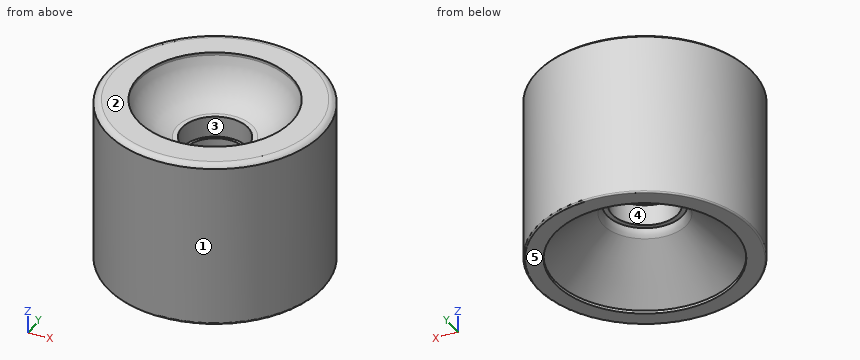
from build123d import *

# Parameters (mm, degrees)
FILLET1_R = 0.5


with BuildPart() as part:
    # Sketch1 → Revolve1 (revolve)
    with BuildSketch(Plane(origin=(0, 0, 0), x_dir=(1, 0, 0), z_dir=(0, 1, 0))):
        with BuildLine():
            Line((36, 56), (36, 1.160679473))
            ThreePointArc((36, 1.160679473), (34.94947687, 0.305750422), (33.63, 0))
            Line((33.63, 0), (25.63, 0))
            Line((25.63, 0), (25.63, 1))
            ThreePointArc((25.63, 1), (20.557422009, 8.606026819), (12.63, 13.16))
            Line((12.63, 13.16), (11, 13.16))
            Line((11, 13.16), (11, 20.16))
            Line((11, 20.16), (10, 20.16))
            Line((10, 20.16), (10, 30.16))
            Line((10, 30.16), (11, 30.16))
            Line((11, 30.16), (11, 37.16))
            Line((11, 37.16), (12.63, 37.16))
            ThreePointArc((12.63, 37.16), (12.964344278, 38.760927271), (13.911484064, 40.094224107))
            Line((13.911484064, 40.094224107), (30, 55))
            Line((30, 55), (30, 56))
            Line((30, 56), (36, 56))
        make_face()
    revolve(axis=Axis((0, 0, 0), (0, 0, -1)))

    # Fillet1
    fillet1_edges = [part.edges().sort_by_distance(p)[0] for p in [
        (-36, 0, -56),
    ]]
    fillet(fillet1_edges, radius=FILLET1_R)


solid = part.part
Here's how the part is built. I have some questions about the finished solid (model axes, mm). Face numbers are marked on the shaded views. A direction names the side the tool comes from. Give positions to 0.01 mm unless a question says otherwise; leave off trailing zeros. Order: outer loops, then holes, each group sorted by start corner. A loop starts at its lowest first (then second) coordinate and runs counter-clockwise, first axis right, second up. Notation, with made-up numbers: M 66.5,-23 L 111.5,-23 A10 ccw 111.5,-16 Z; hole C -24.5,36 d6. An arc over 180 degrees is marked long. Answer as a JSON object with one key per item and string values. Group by question number.
1) We'd pull the mould along Y, two halves only. Please class the marked faces 1, 2 and 3: pulls with the +Y half, pulls with the -Y half, needs draft (parallel to the pull), parting line crosses it, or undercut.
2) Suppose I cut it at A-A, the plane z = -39. Write out the boundary of the cut face in (x, y), plus the area to 3 significant figures.
3) On a 3-axis mill with a long thin cutter (end or side, diameter ignored), from which of +Z, -Z, +X, -X, +Y, -Y can I reach the whole of each face in a straight line? I mean the marked faces 4 and 5. Say none if no direction works.
4) I'm going to push flat-ended pins straight in: pin 1 Ø1.5 at (y, z) = (4, -13.5) entering from -X; pin 2 Ø12 at (y, z) = (18, -22.5) entering from +X; pin 3 Ø4 at (x, z) = (-19, -14) entering from +Y. Where does each tip first touch, or does it pass through?
5) Please list where these lines run through material, in increasing order: L1, parallel to Y at x = 0, z = -0.65; L2, parallel to Y at x = 0, z = -16. Write a range as [from, to].
Results found:
{
 "1": {"face 1": "parting line crosses it", "face 2": "needs draft", "face 3": "undercut"},
 "2": {"outline": "C 0,0 d72; hole C 0,0 d26.16", "area": "3,530 mm²"},
 "3": {"face 4": "-Z", "face 5": "-Z, +X, -X, +Y, -Y"},
 "4": {"pin 1": "x = -35.85", "pin 2": "x = 33.94", "pin 3": "y = 31.73"},
 "5": {"L1": "[-35.49, -25.63], [25.63, 35.49]", "L2": "[-36, -11], [11, 36]"}
}
